from build123d import *

# Parameters (mm, degrees)
SKETCH1_R            = 4
BOSS_EXTRUDE1_DEPTH  = 10
BOSS_EXTRUDE2_DEPTH  = 5
FILLET1_R            = 10
FILLET1_OF_MIRROR1_R = 10


with BuildPart() as part:
    # Sketch1 → Boss-Extrude1 (new body)
    with BuildSketch(Plane.XY):
        with BuildLine():
            Line((-7.444896481, 27.480652594), (-29.444896481, 27.480652594))
            ThreePointArc((-29.444896481, 27.480652594), (-36.515964293, 24.551720406), (-39.444896481, 17.480652594))
            Line((-39.444896481, 17.480652594), (-39.444896481, -19.519347406))
            Line((-39.444896481, -19.519347406), (2.555103519, -19.519347406))
            Line((2.555103519, -19.519347406), (2.555103519, 17.480652594))
            ThreePointArc((2.555103519, 17.480652594), (-0.373828669, 24.551720406), (-7.444896481, 27.480652594))
        make_face()
        with Locations((-18.444896481, -11.019347406)):
            Circle(SKETCH1_R, mode=Mode.SUBTRACT)
    extrude(amount=-BOSS_EXTRUDE1_DEPTH)

    # Sketch2 → Boss-Extrude2 (add)
    with BuildSketch(Plane.ZY.offset(39.444896481)):
        Polygon((0, -19.519347406), (19.519347406, -19.519347406), (0, 0), align=None)
    boss_extrude2 = extrude(amount=-BOSS_EXTRUDE2_DEPTH)

    # Fillet1
    fillet1_edges = [part.edges().sort_by_distance(p)[0] for p in [
        (-36.944896481, 0, 0),
    ]]
    fillet(fillet1_edges, radius=FILLET1_R)

    # Mirror1: Boss-Extrude2 across plane
    add(boss_extrude2.mirror(Plane(origin=(-18.444896481, 0, 0), x_dir=(0, 0, 1), z_dir=(1, 0, 0))))

    # Fillet1 of Mirror1
    fillet1_of_mirror1_edges = [part.edges().sort_by_distance(p)[0] for p in [
        (0.055103519, 0, 0),
    ]]
    fillet(fillet1_of_mirror1_edges, radius=FILLET1_OF_MIRROR1_R)


solid = part.part
For this review, take the finished solid that the model builds, in its own axes (mm). A direction names the side the tool comes from. Round coordinates to 2 decimals unless told otherwise and drop trailing zeros. Write each loop counter-clockwise with the first axis right and the second up, starting at its lowest first coordinate (ties: lowest second). Pieces come first, ordered by that corner, then holes. Notation, with made-up numbers: (56.25, 60.25) -> (105.25, 60.25) arc R4 cw to (105.25, 66.25) -> close; hole circle Ø3 at (29, 11.5). An arc over 180 degrees is marked (long way). Put each result on its own line as item: value.
Q1. The part is to be moulded in two halves that separate along X. For faces 3 (the cylindrical face through (-36.438, 24.629, -4.93)), 4 (the flat face through (-19, 4, -10)), 5 (the flat face through (-19, 4, 0)), say which applies: released by +X, released by -X, zero draft, split by the parting line, or undercut.
Determined:
face 3: released by -X
face 4: zero draft
face 5: undercut
Q2. Consider section C-C on y = -4.5. State the section outline as (x, z) points, and give its area (3 significant figures).
Determined:
outline: (-39.44, -10) -> (2.56, -10) -> (2.56, 4.5) -> (-2.44, 4.5) -> (-2.44, 0) -> (-34.44, 0) -> (-34.44, 4.5) -> (-39.44, 4.5) -> close
area: 465 mm^2
Q3. Consider section B-B on y = -12. State the section outline as (x, z) points, and give its area (3 significant figures).
Determined:
outline: (-39.44, -10) -> (-22.32, -10) -> (-22.32, 0) -> (-34.44, 0) -> (-34.44, 12) -> (-39.44, 12) -> close; (-14.57, -10) -> (2.56, -10) -> (2.56, 12) -> (-2.44, 12) -> (-2.44, 0) -> (-14.57, 0) -> close
area: 462 mm^2
Q4. Consider section D-D on x = -17. State the section outline as (y, z) points, and give its area (3 significant figures).
Determined:
outline: (-19.52, -10) -> (-14.75, -10) -> (-14.75, 0) -> (-19.52, 0) -> close; (-7.29, -10) -> (27.48, -10) -> (27.48, 0) -> (-7.29, 0) -> close
area: 395 mm^2
Q5. Clearance check with flat-ended pins moving along their axes: pin 1 Ø5 at (y, z) = (19.5, 3) entering from -X; pin 2 Ø21 at (x, y) = (-15.5, -4) entering from +Z; pin 3 Ø9 at (x, y) = (-18.44, -11.02) entering from -Z; pin 4 Ø6 at (x, z) = (-5, 14) entering from +Y. State where each tip first meets the part, or that it passes through.
Determined:
pin 1: passes through
pin 2: stops at z = 0
pin 3: stops at z = -10
pin 4: stops at y = -12.43
Q6. Machinability: for faces 1 (the flat face through (-37, -11, 11)), 2 (the flat face through (-34.445, -13, 5)), which of the approach directions +Z, -Z, +X, -X, +Y, -Y give a long, thin tool a straight path to every point of the face, cutting with its end or side? Answer none if there is none.
Determined:
face 1: +Z, +X, -X, +Y
face 2: +Z, +Y, -Y
Q7. Consider section A-A on z = 15. State the section outline as (x, y) points.
Determined:
outline: (-39.44, -19.52) -> (-34.44, -19.52) -> (-34.44, -15) -> (-39.44, -15) -> close; (-2.44, -19.52) -> (2.56, -19.52) -> (2.56, -15) -> (-2.44, -15) -> close
Q8. To check wall thickness, follow L1, parallel to X at y = -12, z = 6; L2, parallel to Z at x = -8, y = 23; L3, parallel to Y at x = -18, z = -2.5. State the ranges of each line that lie inside material, in increasing order. Write a range as [from, to].
Determined:
L1: x = [-39.44, -34.44], [-2.44, 2.56]
L2: z = [-10, 0]
L3: y = [-19.52, -14.99], [-7.04, 27.48]
